```python
from build123d import *

# Parameters (mm, degrees)
IZIM15_R                    = 2
Y_KSEKLIK_EKSTR_ZYON1_DEPTH = 1.5


with BuildPart() as part:
    # Çizim15 → Yükseklik-Ekstrüzyon1 (new body)
    with BuildSketch(Plane(origin=(0, 0, 0), x_dir=(1, 0, 0), z_dir=(0, 1, 0))):
        with BuildLine():
            Line((0, 0), (70, 0))
            Line((70, 0), (97.008301528, 38.571851993))
            Line((97.008301528, 38.571851993), (97.008301528, 127))
            Line((97.008301528, 127), (-15, 127))
            Line((-15, 127), (-15, 55))
            Line((-15, 55), (-15, 50))
            ThreePointArc((-15, 50), (-12.071067812, 42.928932188), (-5, 40))
            Line((-5, 40), (0, 40))
            Line((0, 40), (0, 0))
        make_face()
        with Locations(Location((35.5, 6, 0), (0, 0, 270))):
            Circle(IZIM15_R, mode=Mode.SUBTRACT)
    extrude(amount=Y_KSEKLIK_EKSTR_ZYON1_DEPTH)


solid = part.part
```
Could you check a few things on this model? Use its own coordinates, in mm. Round coordinates to 2 decimals unless told otherwise and drop trailing zeros. Loops run counter-clockwise (first coordinate to the right, second up) from the corner with the lowest first, then second, coordinate; pieces in that order, holes last. Notation, with made-up numbers: M 79,57 L 119,57 A26 ccw 119,94 Z; hole C 68.25,-17.75 d3. An arc over 180 degrees is marked long. Answer as CSV lines item,"result".
1) If I drill on probe 1 along X at (y, z) = (0.4, -6); probe 2 along X at (y, z) = (1.3, -44.5); probe 3 along X at (y, z) = (1, -48.5), over which ranges is the centre line in solid material (lowest first)?
From the geometry:
probe 1,"0 to 33.5, 37.5 to 74.2"
probe 2,"-13.35 to 97.01"
probe 3,"-14.89 to 97.01"
2) Imagine slicing it at A-A on x = 35.5. List the corners of the cut face in (y, z) for me.
From the geometry:
outline,"M 0,-127 L 1.5,-127 L 1.5,-8 L 0,-8 Z; M 0,-4 L 1.5,-4 L 1.5,0 L 0,0 Z"
3) For pin 1 Ø0.8 at (y, z) = (0.5, -24.5) entering from -X, with a flat end and sliding along its axis, tell me the tip position at first contact or that it passes through.
From the geometry:
pin 1,"x = 0"
4) Imagine slicing it at C-C on z = -6. List the corners of the cut face in (x, y) for me, and give its area (3 significant figures).
From the geometry:
outline,"M 0,0 L 33.5,0 L 33.5,1.5 L 0,1.5 Z; M 37.5,0 L 74.2,0 L 74.2,1.5 L 37.5,1.5 Z"
area,"105 mm^2"
5) Imagine slicing it at D-D on z = -19. List the corners of the cut face in (x, y) for me, and give its area (3 significant figures).
From the geometry:
outline,"M 0,0 L 83.3,0 L 83.3,1.5 L 0,1.5 Z"
area,"125 mm^2"
6) Imagine slicing it at B-B on y = 0.25. List the corners of the cut face in (x, z) for me, and give its area (3 significant figures).
From the geometry:
outline,"M -15,-127 L 97.01,-127 L 97.01,-38.57 L 70,0 L 0,0 L 0,-40 L -5,-40 A10 ccw -15,-50 Z; hole C 35.5,-6 d4"
area,"13,100 mm^2"
7) We'd pull the mould along Z, two halves only. Please class faces 1 (the flat face through (40, 0, -64)), 2 (the flat face through (83.32, 0.74, -19.02)), 3 (the cylindrical face through (33.548, 0.74, -6.434)): released by +Z, released by -Z, zero draft, split by the parting line, or undercut.
From the geometry:
face 1,"zero draft"
face 2,"released by +Z"
face 3,"undercut"
